Design review of the part built by this model. Coordinates are the model's own, in mm. A direction names the side the tool comes from. Coordinates: 2 decimals unless noted, no trailing zeros. Write each loop counter-clockwise with the first axis right and the second up, starting at its lowest first coordinate (ties: lowest second). Pieces come first, ordered by that corner, then holes.
Q1. Insertion check: pin 1 (1.5 mm diameter, centred on x = -1, y = 1.5, fed in from -Z); pin 2 (1.6 mm diameter, centred on x = 0, y = 0, fed in from +Z). Each pin has a flat end and moves straight along its axis. Give the tip position at first contact, or say it passes through.
Q2. Machinability: for faces 4 (the flat face through (-0.4, -1.1, 0)), 5 (the flat face through (0, 0, -3)), 6 (the flat face through (0, 0, 37)), which of the approach directions +Z, -Z, +X, -X, +Y, -Y give a long, thin tool a straight path to every point of the face, cutting with its end or side? Answer none if there is none.
Q3. Take a section at A-A (y = 0). Give the boundary of the cut face in (x, z), and give its area (3 significant figures).
Q4. For probe 1 along Y at (x, z) = (0, 37.9); probe 2 along Y at (x, z) = (0.4, 19); probe 3 along Z at (x, y) = (-1.25, -0.2), list the stretches that pass through material, from the lowest coordinate up.
Q5. Mouldability with a two-part tool opening along Y and no side actions: class faces 1 (the flat face through (-0.4, -1.1, 40)), 2 (the flat face through (-0.76, 1.293, 19.72)), 3 (the cylindrical face through (0, -1, 39)) as pulls with the +Y half, pulls with the -Y half, needs draft (parallel to the pull), parting line crosses it, or undercut.
Q6. Take a section at B-B (z = 15). Give the boundary of the cut face in (x, y).
Autodesk Inventor part; units mm, degrees
ref_plane "YZ Plane" through (0, 0, 0) normal (1, 0, 0) x (0, 1, 0)
ref_plane "XZ Plane" through (0, 0, 0) normal (0, 1, 0) x (-1, 0, 0)
ref_plane "XY Plane" through (0, 0, 0) normal (0, 0, 1) x (1, 0, 0)
sketch "Sketch1" plane through (0, 0, 0) normal (0, 0, 1) x (1, 0, 0)
  line L0 (0, 1.7321) -> (1.5, 0.866)
  line L1 (1.5, 0.866) -> (1.5, -0.866)
  line L2 (1.5, -0.866) -> (0, -1.7321)
  line L3 (0, -1.7321) -> (-1.5, -0.866)
  line L4 (-1.5, -0.866) -> (-1.5, 0.866)
  line L5 (-1.5, 0.866) -> (0, 1.7321)
  point P0 (0, 0)
  point P1 (0, 0)
  dimension "d0" = 3
extrude "Extrusion1" add sketch "Sketch1" along normal blind 40
sketch "Sketch2" plane through (0, 0, 40) normal (0, 0, 1) x (1, 0, 0)
  circle A0 centre (0, 0) radius 1
  dimension "d3" = 2
extrude "Extrusion2" cut sketch "Sketch2" against normal blind 3
sketch "Sketch3" plane through (0, 0, 0) normal (0, 0, -1) x (-1, 0, 0)
  circle A0 centre (0, 0) radius 1
extrude "Extrusion3" add sketch "Sketch3" along normal blind 3
thread "Thread1"
thread "Thread2"
properties part number "M2_40mm_standoff"
Response:
1. pin 1: stops at z = 0
1. pin 2: stops at z = 37
2. face 4: -Z
2. face 5: -Z, +X, -X, +Y, -Y
2. face 6: +Z
3. outline: (-1.5, 0) - (-1, 0) - (-1, -3) - (1, -3) - (1, 0) - (1.5, 0) - (1.5, 40) - (1, 40) - (1, 37) - (-1, 37) - (-1, 40) - (-1.5, 40) - close
3. area: 120 mm2
4. probe 1: y = -1.73 to -1, 1 to 1.73
4. probe 2: y = -1.5 to 1.5
4. probe 3: z = 0 to 40
5. face 1: needs draft
5. face 2: pulls with the +Y half
5. face 3: undercut
6. outline: (-1.5, -0.87) - (0, -1.73) - (1.5, -0.87) - (1.5, 0.87) - (0, 1.73) - (-1.5, 0.87) - close
